from build123d import *


with BuildPart() as part:
    # Esquisse1 → Révolution1 (revolve)
    with BuildSketch(Plane.XY):
        with BuildLine():
            Line((12.75, -3.2), (12.75, -6.2))
            Line((12.75, -6.2), (1.5, -6.2))
            Line((1.5, -6.2), (1.5, -10.7))
            Line((1.5, -10.7), (0, -10.7))
            Line((0, -10.7), (0, 6))
            ThreePointArc((0, 6), (2.449489743, 5.477225575), (4.472135955, 4))
            Line((4.472135955, 4), (6.472135955, 4))
            Line((6.472135955, 4), (12.75, -3.2))
        make_face()
    revolve(axis=Axis((0, 6, 0), (0, -1, 0)))


solid = part.part
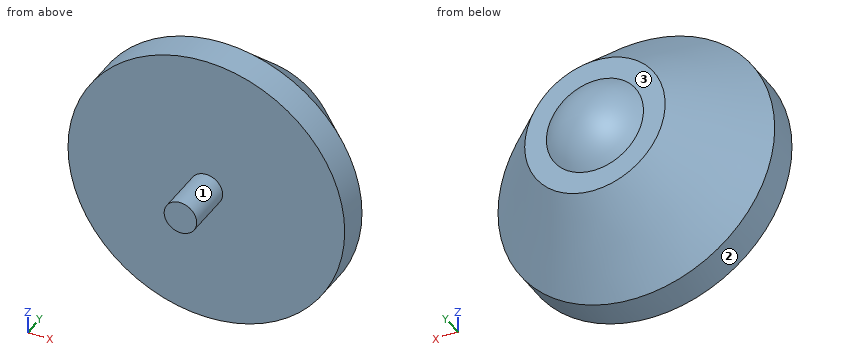
Source: CAD feature listing. Evaluate the final solid. Frame: model axes, mm. Face numbers are marked on the shaded views. A direction names the side the tool comes from. Round coordinates to 2 decimals unless told otherwise and drop trailing zeros. Loops run counter-clockwise (first coordinate to the right, second up) from the corner with the lowest first, then second, coordinate; pieces in that order, holes last.
Q1. Ray query, line 1 (Y direction, x = -1.5, z = 5); line 2 (Z direction, x = 1.5, y = 1); line 3 (X direction, y = -5.25, z = -4.25). Return the intervals inside material, ascending.
Q2. Section A-A, the plane z = 0. Return loops of the section in (x, y).
Q3. First-contact query: P1, Ø8, axis at x = 1, y = -2.5, coming from the -Z side; P2, Ø4, axis at x = -2.5, z = 2.5, coming from the +Y side; P3, Ø5, axis at x = 4.5, y = -7, coming from the -Z side; P4, Ø12, axis at x = -9.5, z = -8, coming from the -Y side. Flat tips, straight axial feed; report the tip coordinate or a pass-through.
Q4. Access query for the marked faces 1, 2 and 3. Directions: +Z, -Z, +X, -X, +Y, -Y. A direction counts if a zero-diameter tool reaches every point of the face in a straight line with its end or side. Return the directions, or none.
Q5. Section B-B, the plane y = -5. Return loops of the section in (x, z).
Q6. Section C-C, the plane y = -9.5. Return loops of the section in (x, z), plus the area to 3 significant figures.
Solutions:
1. line 1: y = -6.2 to 4
1. line 2: z = -8.96 to 8.96
1. line 3: x = -12.02 to 12.02
2. outline: (-12.75, -6.2) - (-1.5, -6.2) - (-1.5, -10.7) - (1.5, -10.7) - (1.5, -6.2) - (12.75, -6.2) - (12.75, -3.2) - (6.47, 4) - (4.47, 4) arc R6 ccw to (-4.47, 4) - (-6.47, 4) - (-12.75, -3.2) - close
3. P1: stops at z = -12.75
3. P2: stops at y = 5.8
3. P3: stops at z = -12.57
3. P4: stops at y = -6.2
4. face 1: -Y
4. face 2: +Y, -Y
4. face 3: +Y
5. outline: circle Ø25.5 at (0, 0)
6. outline: circle Ø3 at (0, 0)
6. area: 7.07 mm2
